Design review of the part built by this model. Coordinates are the model's own, in mm. A direction names the side the tool comes from. Coordinates: 2 decimals unless noted, no trailing zeros. Loops run counter-clockwise (first coordinate to the right, second up) from the corner with the lowest first, then second, coordinate; pieces in that order, holes last.
Q1. Add section B-B on x = 11.5. Give the boundary of the cut face in (y, z), and give its area (3 significant figures).
Q2. Add section A-A on z = 7.5. Give the boundary of the cut face in (x, y) (3 decimals).
Q3. Draft analysis for pull direction X (two halves, no side actions). For faces 1 (the face through (9.525, 38, -1)), 2 (the face through (16, 38, 11.112)), 3 (the face through (-9.792, 21.914, 0.178)), state which applies: released by +X, released by -X, zero draft, split by the parting line, or undercut.
Q4. Wall thickness on probe 1 along X at (y, z) = (-39, -7.25) (3 decimals); probe 2 along Y at (x, z) = (20, -9.25); probe 3 along Y at (x, z) = (4, 10): over which ranges is each line inside the solid? List them lowest first.
Q5. Machinability: for faces 4 (the face through (16, 31.75, -1)), 5 (the face through (-4, 0, 0)), 6 (the face through (6, 11, 12.7)), which of the approach directions +Z, -Z, +X, -X, +Y, -Y give a long, thin tool a straight path to every point of the face, cutting with its end or side? Answer none if there is none.
Q6. Add section C-C on y = -24.5. Give the boundary of the cut face in (x, z) (3 decimals).
Q7. For P1, Ø4, axis at x = 0.5, z = -1.5, coming from the +Y side; P2, Ø4, axis at x = 19, z = 2, coming from the +Y side; P3, Ø1.5, axis at x = 3, z = -8, coming from the -Y side, all flat-tipped, find the tip position at first contact; note any pin that passes through.
Q8. Add section D-D on x = -24. Give the boundary of the cut face in (y, z), and give its area (3 significant figures).
```python
from build123d import *

# Parameters (mm, degrees)
BOSS_EXTRUDE1_DEPTH = 12.7
SKETCH2_W           = 12.7
SKETCH2_H           = 12.7
CUT_EXTRUDE1_DEPTH  = 23.8125


with BuildPart() as part:
    # Sketch1 → Boss-Extrude1 (new, symmetric)
    with BuildSketch(Plane.XY):
        Polygon((19.05, -50.8), (19.05, 0), (-28.575, 0), (9.525, 44.45), (22.225, 44.45), (22.225, 31.75), (22.225, -50.8), align=None)
    extrude(amount=BOSS_EXTRUDE1_DEPTH, both=True)

    # Sketch2 → Cut-Extrude1 (cut)
    with BuildSketch(Plane(origin=(0, 0, -12.7), x_dir=(-1, 0, 0), z_dir=(0, 0, -1))):
        with Locations((-15.875, 38.1)):
            Rectangle(SKETCH2_W, SKETCH2_H)
    extrude(amount=-CUT_EXTRUDE1_DEPTH, mode=Mode.SUBTRACT)


solid = part.part
```
Entries:
1. outline: (0, -12.7) - (31.75, -12.7) - (31.75, 11.11) - (44.45, 11.11) - (44.45, 12.7) - (0, 12.7) - close
1. area: 827 mm2
2. outline: (-28.575, 0) - (19.05, 0) - (19.05, -50.8) - (22.225, -50.8) - (22.225, 31.75) - (9.525, 31.75) - (9.525, 44.45) - close
3. face 1: released by +X
3. face 2: zero draft
3. face 3: released by -X
4. probe 1: x = 19.05 to 22.225
4. probe 2: y = -50.8 to 31.75
4. probe 3: y = 0 to 38
5. face 4: -Z, +X, +Y
5. face 5: +Z, -Z, -X, -Y
5. face 6: +Z, +X, -X, +Y, -Y
6. outline: (19.05, -12.7) - (22.225, -12.7) - (22.225, 12.7) - (19.05, 12.7) - close
7. P1: stops at y = 36.25
7. P2: stops at y = 31.75
7. P3: stops at y = 0
8. outline: (0, -12.7) - (5.34, -12.7) - (5.34, 12.7) - (0, 12.7) - close
8. area: 136 mm2
